The drawing under review shows one solid part. Ordinate dimensions are in mm from its lowest x, y, z. A direction names the side the tool comes from. Round coordinates to 2 decimals unless told otherwise and drop trailing zeros. Write each loop counter-clockwise with the first axis right and the second up, starting at its lowest first coordinate (ties: lowest second). Pieces come first, ordered by that corner, then holes. Notation, with made-up numbers: (2, -1) -> (38, -1) arc R31 cw to (38, 26) -> close; hole circle Ø5 at (-26, -0.75). An arc over 180 degrees is marked (long way). Answer in a Markdown table with one row per item.
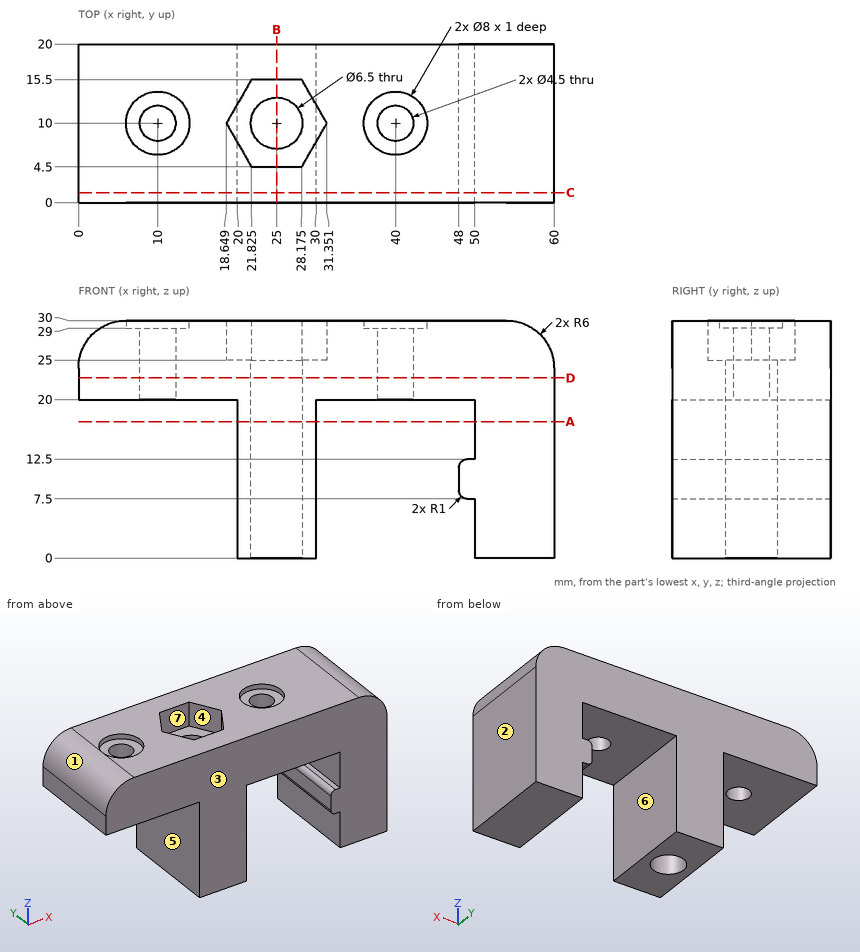
1) Clearance check with flat-ended pins moving along their axes: pin 1 Ø6 at (x, z) = (45.5, 13.5) entering from -Y; pin 2 Ø10.5 at (x, y) = (25, 10) entering from -Z; pin 3 Ø6.5 at (x, y) = (40, 10) entering from +Z; pin 4 Ø9 at (x, y) = (10, 10) entering from -Z. State where each tip first meets the part, or that it passes through.
Solved:
| item | result |
|---|---|
| pin 1 | through |
| pin 2 | z = 0 |
| pin 3 | z = 29 |
| pin 4 | z = 20 |
2) For line 1 (X direction, y = 8.5, z = 2.75); line 2 (X direction, y = 8, z = 10); line 3 (Y direction, x = 25, z = 6.5), list the stretches that pass through material, from the lowest coordinate up. Write a range as [from, to].
Solved:
| item | result |
|---|---|
| line 1 | [20, 22.12], [27.88, 30], [50, 60] |
| line 2 | [20, 22.44], [27.56, 30], [48, 60] |
| line 3 | [0, 6.75], [13.25, 20] |
3) For the marked faces 5, 6 and 7, list the 3-axis set-ups (+Z, -Z, +X, -X, +Y, -Y) from which the entire face can be reached by the end or side of a thin tool; tool diameter is ignored.
Solved:
| item | result |
|---|---|
| face 5 | -Z, -X, +Y, -Y |
| face 6 | -Z, +Y, -Y |
| face 7 | +Z |
4) Consider section C-C on y = 1.25. State the section outline as (x, z) points, then the cut area to 3 significant figures.
Solved:
| item | result |
|---|---|
| outline | (0, 20) -> (20, 20) -> (20, 0) -> (30, 0) -> (30, 20) -> (50, 20) -> (50, 12.5) -> (49, 12.5) arc R1 ccw to (48, 11.5) -> (48, 8.5) arc R1 ccw to (49, 7.5) -> (50, 7.5) -> (50, 0) -> (60, 0) -> (60, 24) arc R6 ccw to (54, 30) -> (6, 30) arc R6 ccw to (0, 24) -> close |
| area | 994 mm² |
5) Consider section A-A on z = 17.25. State the section outline as (x, y) points.
Solved:
| item | result |
|---|---|
| outline | (20, 0) -> (30, 0) -> (30, 20) -> (20, 20) -> close; (50, 0) -> (60, 0) -> (60, 20) -> (50, 20) -> close; hole circle Ø6.5 at (25, 10) |
6) Consider section D-D on z = 22.75. State the section outline as (x, y) points.
Solved:
| item | result |
|---|---|
| outline | (0, 0) -> (60, 0) -> (60, 20) -> (0, 20) -> close; hole circle Ø4.5 at (10, 10); hole circle Ø6.5 at (25, 10); hole circle Ø4.5 at (40, 10) |
7) Mouldability with a two-part tool opening along X and no side actions: class the marked faces 1, 2, 3 and 4 as pulls with the +X half, pulls with the -X half, needs draft (parallel to the pull), parting line crosses it, or undercut.
Solved:
| item | result |
|---|---|
| face 1 | pulls with the -X half |
| face 2 | pulls with the +X half |
| face 3 | needs draft |
| face 4 | undercut |
8) Consider section B-B on x = 25. State the section outline as (y, z) points.
Solved:
| item | result |
|---|---|
| outline | (0, 0) -> (6.75, 0) -> (6.75, 25) -> (4.5, 25) -> (4.5, 30) -> (0, 30) -> close; (13.25, 0) -> (20, 0) -> (20, 30) -> (15.5, 30) -> (15.5, 25) -> (13.25, 25) -> close |
